from build123d import *

# Parameters (mm, degrees)
OTW_R_GWINTOWANY_M81_D     = 6.8
OTW_R_GWINTOWANY_M81_DEPTH = 12.25
OTW_R_GWINTOWANY_M81_TIP   = 2.042926105
SFAZOWANIE1_SIZE           = 1
SFAZOWANIE2_SIZE           = 1


with BuildPart() as part:
    # Szkic1 → Obrót1 (revolve)
    with BuildSketch(Plane.XY, mode=Mode.PRIVATE) as obr_t1_sk:
        Polygon((-133.522258266, 0), (-133.522258266, 15), (-106.522258266, 15), (-106.522258266, 14), (-103.522258266, 14), (-103.522258266, 25), (0.919675372, 25), (6.477741734, 15), (224.810321825, 15), (226.477741734, 12), (326.477741734, 12), (326.477741734, 0), align=None)
    revolve(obr_t1_sk.sketch.rotate(Axis((-73.178837214, 0, 0), (1, 0, 0)), 90), axis=Axis((-73.178837214, 0, 0), (1, 0, 0)))

    # Otwór gwintowany M81
    with Locations(Plane.ZY.offset(133.522258266)):
        with Locations((0, 0)):
            Hole(OTW_R_GWINTOWANY_M81_D / 2, depth=OTW_R_GWINTOWANY_M81_DEPTH)
            with Locations((0, 0, -(OTW_R_GWINTOWANY_M81_DEPTH + OTW_R_GWINTOWANY_M81_TIP / 2))):  # 118° drill point
                Cone(0, OTW_R_GWINTOWANY_M81_D / 2, OTW_R_GWINTOWANY_M81_TIP, mode=Mode.SUBTRACT)

    # Sfazowanie1
    sfazowanie1_edges = [part.edges().sort_by_distance(p)[0] for p in [
        (-133.522258266, 0, -15),
    ]]
    chamfer(sfazowanie1_edges, length=SFAZOWANIE1_SIZE)

    # Sfazowanie2
    sfazowanie2_edges = [part.edges().sort_by_distance(p)[0] for p in [
        (326.477741734, 0, -12),
    ]]
    chamfer(sfazowanie2_edges, length=SFAZOWANIE2_SIZE)


solid = part.part
Source: CAD feature listing. Evaluate the final solid. Frame: model axes, mm. A direction names the side the tool comes from. Round coordinates to 2 decimals unless told otherwise and drop trailing zeros. Loops run counter-clockwise (first coordinate to the right, second up) from the corner with the lowest first, then second, coordinate; pieces in that order, holes last. Notation, with made-up numbers: M 23,1 L 64,1 A19 cw 64,36 Z; hole C 21,38.5 d1. An arc over 180 degrees is marked long. Answer as CSV lines item,"result".
Q1. Reachability of faces 1 (the face through (276.671, -3.604, 11.446)), 2 (the face through (-119.34, -12.65, 8.06)), 3 (the face through (326.478, 0, 0)) from +Z, -Z, +X, -X, +Y, -Y: full face, straight path, thin tool, end or side. Return the list, or none.
Verdict:
face 1,"+X"
face 2,"-X"
face 3,"+Z, -Z, +X, +Y, -Y"
Q2. Cut plane A-A (x = 60). Return the cut outline in (y, z), plus the area to 3 significant figures.
Verdict:
outline,"C 0,0 d30"
area,"707 mm^2"
Q3. Cut plane B-B (x = -52.5). Return the cut outline in (y, z).
Verdict:
outline,"C 0,0 d50"
Q4. Pull-direction query (X, two-part tool) for faces 4 (the face through (-105, 12.4, 6.5)), 5 (the face through (6.21, -4.65, 14.77)), 6 (the face through (117.17, -12.65, 8.06)); classes: +X half, -X half, draft (parallel to the pull), parting line (faces both ways), or undercut.
Verdict:
face 4,"undercut"
face 5,"+X half"
face 6,"draft"
Q5. Contact query for flat-ended pins moving along their axis: pin 1 (1.5 mm diameter, centred on y = -0.5, z = 17, fed in from -X); pin 2 (1.5 mm diameter, centred on x = -72.5, z = -19, fed in from -Y); pin 3 (4 mm diameter, centred on x = 16, z = -11, fed in from -Y). Output: stop coordinate, or through.
Verdict:
pin 1,"stops at x = -103.52"
pin 2,"stops at y = -17.09"
pin 3,"stops at y = -12"
Q6. Line query: line 1 along Y through (x, z) = (-127.75, 0); line 2 along X through (y, z) = (20, 4); line 3 along X through (y, z) = (-15, -1). Output: solid intervals per line, ascending.
Verdict:
line 1,"y = -15 to -3.4, 3.4 to 15"
line 2,"x = -103.52 to 3.48"
line 3,"x = -103.52 to 6.46"
